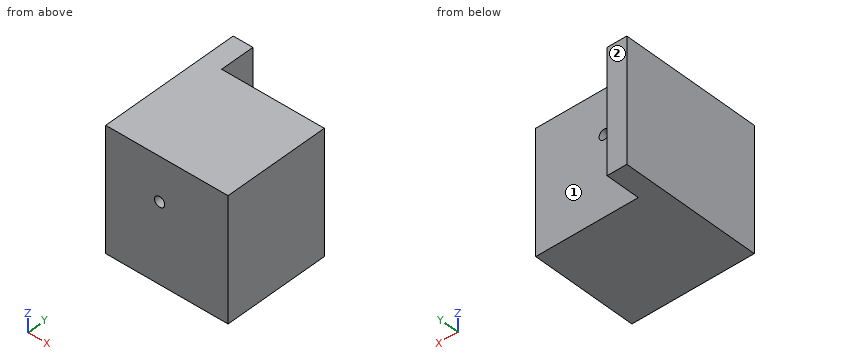
```python
from build123d import *

# Parameters (mm, degrees)
F1_DEPTH = 50.8
F3_D     = 4.2


with BuildPart() as f1:
    # F0 (on Top) → F1 (new body)
    with BuildSketch(Plane.XY):
        Polygon((-108.0991402268, 14.2310541123), (-116.2496432662, 14.2310541123), (-116.2496432662, -43.835349381), (-65.739735961, -43.835349381), (-65.739735961, 0), (-108.0991402268, 0), align=None)
    extrude(amount=F1_DEPTH)

    # F3 (through all)
    with Locations(Plane.XZ.offset(43.835349381)):
        with Locations((-93.9946100116, 32.7801704407)):
            Hole(F3_D / 2)


solid = f1.part
```
Can you work these out from the model? Positions are in its coordinate system, mm. Face numbers are marked on the shaded views. A direction names the side the tool comes from. Give positions to 0.01 mm unless a question says otherwise; leave off trailing zeros. Loops run counter-clockwise (first coordinate to the right, second up) from the corner with the lowest first, then second, coordinate; pieces in that order, holes last. Notation, with made-up numbers: M -20.75,74 L 35.25,74 A13 cw 35.25,98 Z; hole C -14.75,38.5 d5. An arc over 180 degrees is marked long. One line per question, with ' | ' between items. Start each with the question number.
Q1. If we section it at C-C (y = 1.5): Please give me the cut outline in (x, z), plus the area to 3 significant figures.
Q2. If we section it at B-B (z = 6.5): Please give me the cut outline in (x, y), plus the area to 3 significant figures.
Q3. If I drill on line 1 (Y direction, x = -104, z = 21.5); line 2 (Z direction, x = -93, y = -26), over which ranges is the centre line in solid material (lowest first)? Write a range as from..to.
Q4. If we section it at D-D (x = -87): Please give me the cut outline in (y, z), plus the area to 3 significant figures.
Q5. If we section it at A-A (x = -94): Please give me the cut outline in (y, z).
Q6. For pin 1 Ø12.5 at (x, z) = (-97.5, 23) entering from +Y; pin 2 Ø4.5 at (y, z) = (5.5, 33.5) entering from +X, each with a flat end and sliding along its axis, tell me the tip position at first contact or that it passes through.
Q7. For the marked faces 1 and 2, which set-ups out of +Z, -Z, +X, -X, +Y, -Y let a thin tool reach every point of the face, with its end or its side?
Computed:
1) outline: M -116.25,0 L -108.1,0 L -108.1,50.8 L -116.25,50.8 Z | area: 414 mm²
2) outline: M -116.25,-43.84 L -65.74,-43.84 L -65.74,0 L -108.1,0 L -108.1,14.23 L -116.25,14.23 Z | area: 2,330 mm²
3) line 1: y = -43.84..0 | line 2: z = 0..30.93, 34.63..50.8
4) outline: M -43.84,0 L 0,0 L 0,50.8 L -43.84,50.8 Z | area: 2,230 mm²
5) outline: M -43.84,0 L 0,0 L 0,30.68 L -43.84,30.68 Z; M -43.84,34.88 L 0,34.88 L 0,50.8 L -43.84,50.8 Z
6) pin 1: stops at y = 0 | pin 2: stops at x = -108.1
7) face 1: +Z, -Z, +X, +Y | face 2: +Z, -Z, +X, -X, +Y
